CAD build for the part. Positions are in the model's coordinates, mm. Face numbers are marked on the shaded views. A direction names the side the tool comes from. Coordinates: 2 decimals unless noted, no trailing zeros. Order: outer loops, then holes, each group sorted by start corner. A loop starts at its lowest first (then second) coordinate and runs counter-clockwise, first axis right, second up. Notation, with made-up numbers: M -36,-32 L 4,-32 A27 ccw 4,-14 Z; hole C 20,57 d11. An arc over 180 degrees is marked long. Write item = value, one per line.
from build123d import *

# Parameters (mm, degrees)
SKETCH_1_W          = 450
SKETCH_1_H          = 450
EXTRUDE_1_DEPTH     = 250
SKETCH_2_W          = 180
SKETCH_2_H          = 240
CUT_EXTRUDE_1_DEPTH = 50
SKETCH_3_W          = 110
SKETCH_3_H          = 100
CUT_EXTRUDE_2_DEPTH = 50
SKETCH_4_W          = 8
SKETCH_4_H          = 12
CUT_EXTRUDE_3_DEPTH = 20
SKETCH_5_W          = 8
SKETCH_5_H          = 12
CUT_EXTRUDE_4_DEPTH = 20
SKETCH_6_W          = 20
SKETCH_6_H          = 20
EXTRUDE_2_DEPTH     = 600
SKETCH_7_W          = 20
SKETCH_7_H          = 20
EXTRUDE_3_DEPTH     = 600


with BuildPart() as part:
    # 草图1 → 凸台-拉伸1 (new body)
    with BuildSketch(Plane(origin=(0, 0, 0), x_dir=(1, 0, 0), z_dir=(0, 1, 0))):
        Rectangle(SKETCH_1_W, SKETCH_1_H)
    extrude(amount=EXTRUDE_1_DEPTH)

    # 草图2 → 切除-拉伸1 (cut)
    with BuildSketch(Plane(origin=(0, 250, 0), x_dir=(1, 0, 0), z_dir=(0, 1, 0))):
        with Locations((0, 45)):
            Rectangle(SKETCH_2_W, SKETCH_2_H)
    extrude(amount=-CUT_EXTRUDE_1_DEPTH, mode=Mode.SUBTRACT)

    # 草图3 → 切除-拉伸2 (cut)
    with BuildSketch(Plane(origin=(0, 250, 0), x_dir=(1, 0, 0), z_dir=(0, 1, 0))):
        with Locations((-170, 175)):
            Rectangle(SKETCH_3_W, SKETCH_3_H)
        with Locations((170, 175)):
            Rectangle(SKETCH_3_W, SKETCH_3_H)
    extrude(amount=-CUT_EXTRUDE_2_DEPTH, mode=Mode.SUBTRACT)

    # 草图4 → 切除-拉伸3 (cut)
    with BuildSketch(Plane(origin=(0, 0, -225), x_dir=(-1, 0, 0), z_dir=(0, 0, -1))):
        with Locations((-101, 236)):
            Rectangle(SKETCH_4_W, SKETCH_4_H)
        with Locations((101, 236)):
            Rectangle(SKETCH_4_W, SKETCH_4_H)
    extrude(amount=-CUT_EXTRUDE_3_DEPTH, mode=Mode.SUBTRACT)

    # 草图5 → 切除-拉伸4 (cut)
    with BuildSketch(Plane(origin=(0, 0, -125), x_dir=(-1, 0, 0), z_dir=(0, 0, -1))):
        with Locations((216, 236)):
            Rectangle(SKETCH_5_W, SKETCH_5_H)
    extrude(amount=-CUT_EXTRUDE_4_DEPTH, mode=Mode.SUBTRACT)

    # 草图6 → 凸台-拉伸2 (add)
    with BuildSketch(Plane.XZ):
        with Locations((-215, 215)):
            Rectangle(SKETCH_6_W, SKETCH_6_H)
    extrude(amount=-EXTRUDE_2_DEPTH)

    # 草图7 → 凸台-拉伸3 (add)
    with BuildSketch(Plane.XY.offset(225)):
        with Locations((-215, 10)):
            Rectangle(SKETCH_7_W, SKETCH_7_H)
    extrude(amount=-EXTRUDE_3_DEPTH)


solid = part.part
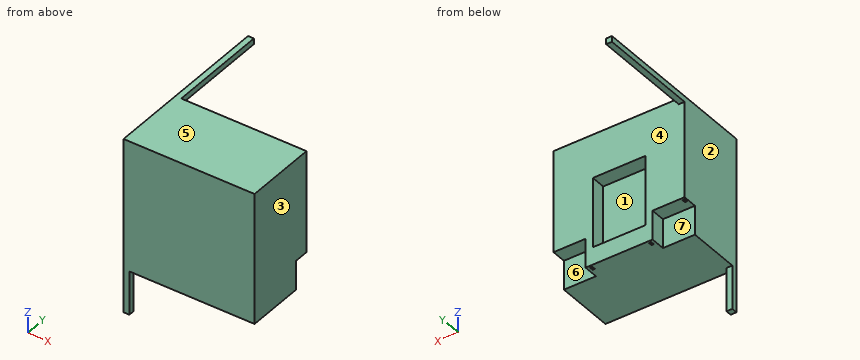
(1) Wall check: line 1 (Y direction, x = -12, z = -104); line 2 (Z direction, x = 14, y = 126.5); line 3 (Y direction, x = -24, z = -211.5). Give the ranges that are in metal, low to high. Write a range as from..to.
Evaluation:
line_1 = 0..200
line_2 = -225..225
line_3 = 0..250
(2) Pin check, flat tips, straight feed: pin 1 Ø9 at (x, z) = (99, -210.5) entering from +Y; pin 2 Ø15 at (x, y) = (-153.5, 233.5) entering from -Z; pin 3 Ø22 at (x, z) = (-216.5, -273) entering from +Y; pin 4 Ø8 at (x, z) = (139.5, 72) entering from -Y. Stop position of each tip, or through.
Evaluation:
pin_1 = 250
pin_2 = -125
pin_3 = 20
pin_4 = 0
(3) Slice it at A-A, the plane y = 216. Write the cut outline in (x, z), then the cut area to 3 significant figures.
Evaluation:
outline = M -225,-125 L -115,-125 L -115,-225 L 115,-225 L 115,-125 L 225,-125 L 225,225 L -225,225 Z; hole M -90,-165 L 90,-165 L 90,75 L -90,75 Z
area = 137,000 mm²
(4) Slice it at C-C, the plane z = -10. Write the cut outline in (x, y), then the cut area to 4 significant figures.
Evaluation:
outline = M -225,0 L 225,0 L 225,250 L 90,250 L 90,200 L -90,200 L -90,250 L -225,250 Z
area = 103,500 mm²
(5) Tool access for the marked faces 5, 6 and 7: list every direction of +Z, -Z, +X, -X, +Y, -Y with a clear straight run to the whole face (end or side of a thin tool).
Evaluation:
face_5 = +Z, +X, -X, +Y, -Y
face_6 = -Z, +X, +Y
face_7 = -Z, -X, +Y
(6) Slice it at D-D, the plane y = 124. Write the cut outline in (x, z), then the cut area to 4 significant figures.
Evaluation:
outline = M -225,-225 L 225,-225 L 225,225 L -225,225 Z
area = 202,500 mm²
(7) Slice it at B-B, the plane x = 58. Write the cut outline in (y, z), then the cut area to 4 significant figures.
Evaluation:
outline = M 0,-225 L 250,-225 L 250,-165 L 200,-165 L 200,75 L 250,75 L 250,225 L 0,225 Z
area = 100,500 mm²
(8) Pull direction X, two halves, no side cores. Call the marked faces 1, 2, 3 and 4: +X half, -X half, draft (parallel to the pull), parting line (faces both ways), or undercut.
Evaluation:
face_1 = undercut
face_2 = -X half
face_3 = +X half
face_4 = draft
